Verification items for the finished model (mm, model axes). Face numbers are marked on the shaded views. A direction names the side the tool comes from. Coordinates: 2 decimals unless noted, no trailing zeros. Order: outer loops, then holes, each group sorted by start corner. A loop starts at its lowest first (then second) coordinate and runs counter-clockwise, first axis right, second up. Notation, with made-up numbers: (-19.5, 13.25) -> (-14.5, 13.25) arc R32 ccw to (-14.5, 44.25) -> close; hole circle Ø3 at (36.25, 44.25). An arc over 180 degrees is marked (long way). Use CSV: the item, a comma, the result in double quotes. Start each with the question number.
1) Go/stop test with flat-tipped pins: pin 1 (2 mm diameter, centred on x = 38.5, y = 0, fed in from -Z); pin 2 (1.5 mm diameter, centred on x = 28, y = 1.5, fed in from +Z); pin 3 (0.8 mm diameter, centred on y = 0, z = 0, fed in from -X). Record where each tip stops, or that it passes through.
2) Sectioned sample at A-A on z = 0. Record the boundary of the cut face in (x, y).
3) Sectioned sample at B-B on x = 19. Record the boundary of the cut face in (y, z), then the cut area to 3 significant figures.
4) Scan lines: line 1 along X through (y, z) = (-2.45, 0.45); line 2 along Z through (x, y) = (23, 0.1); line 3 along X through (y, z) = (0.15, 0.55). Record each from-to range of solid material in increasing order.
5) Tool access check on the marked faces 1 and 2. Record the directions out of +Z, -Z, +X, -X, +Y, -Y that give a thin tool (end or side, any length) a straight path to the whole face; none if there is none.
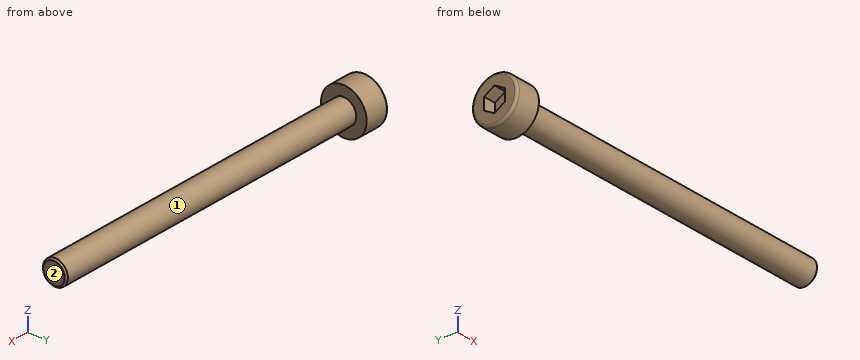
from build123d import *

# Parameters (mm, degrees)
SCHNITT_LINEAR_AUSTRAGEN1_DEPTH = 1.5


with BuildPart() as part:
    # Skizze1 → Rotation1 (revolve)
    with BuildSketch(Plane.XY):
        with BuildLine():
            Line((0, 0), (0, 2.45))
            ThreePointArc((0, 2.45), (0.087867966, 2.662132034), (0.3, 2.75))
            Line((0.3, 2.75), (3, 2.75))
            Line((3, 2.75), (3, 1.5))
            Line((3, 1.5), (42.8, 1.5))
            Line((42.8, 1.5), (43, 1.3))
            Line((43, 1.3), (43, 0))
            Line((43, 0), (0, 0))
        make_face()
    revolve(axis=Axis((0, 0, 0), (1, 0, 0)))

    # Skizze2 → Schnitt-Linear austragen1 (cut)
    with BuildSketch(Plane.ZY):
        Polygon((1.443375673, 0), (0.721687836, 1.25), (-0.721687836, 1.25), (-1.443375673, 0), (-0.721687836, -1.25), (0.721687836, -1.25), align=None)
    extrude(amount=-SCHNITT_LINEAR_AUSTRAGEN1_DEPTH, mode=Mode.SUBTRACT)


solid = part.part
Answers follow:
1,pin 1,"stops at z = -1.5"
1,pin 2,"stops at z = 1.3"
1,pin 3,"stops at x = 1.5"
2,outline,"(0, -2.45) arc R0.3 ccw to (0.3, -2.75) -> (3, -2.75) -> (3, -1.5) -> (42.8, -1.5) -> (43, -1.3) -> (43, 1.3) -> (42.8, 1.5) -> (3, 1.5) -> (3, 2.75) -> (0.3, 2.75) arc R0.3 ccw to (0, 2.45) -> (0, 1.25) -> (1.5, 1.25) -> (1.5, -1.25) -> (0, -1.25) -> close"
3,outline,"circle Ø3 at (0, 0)"
3,area,"7.07 mm²"
4,line 1,"x = 0 to 3"
4,line 2,"z = -1.5 to 1.5"
4,line 3,"x = 1.5 to 43"
5,face 1,"+X"
5,face 2,"+Z, -Z, +X, +Y, -Y"
